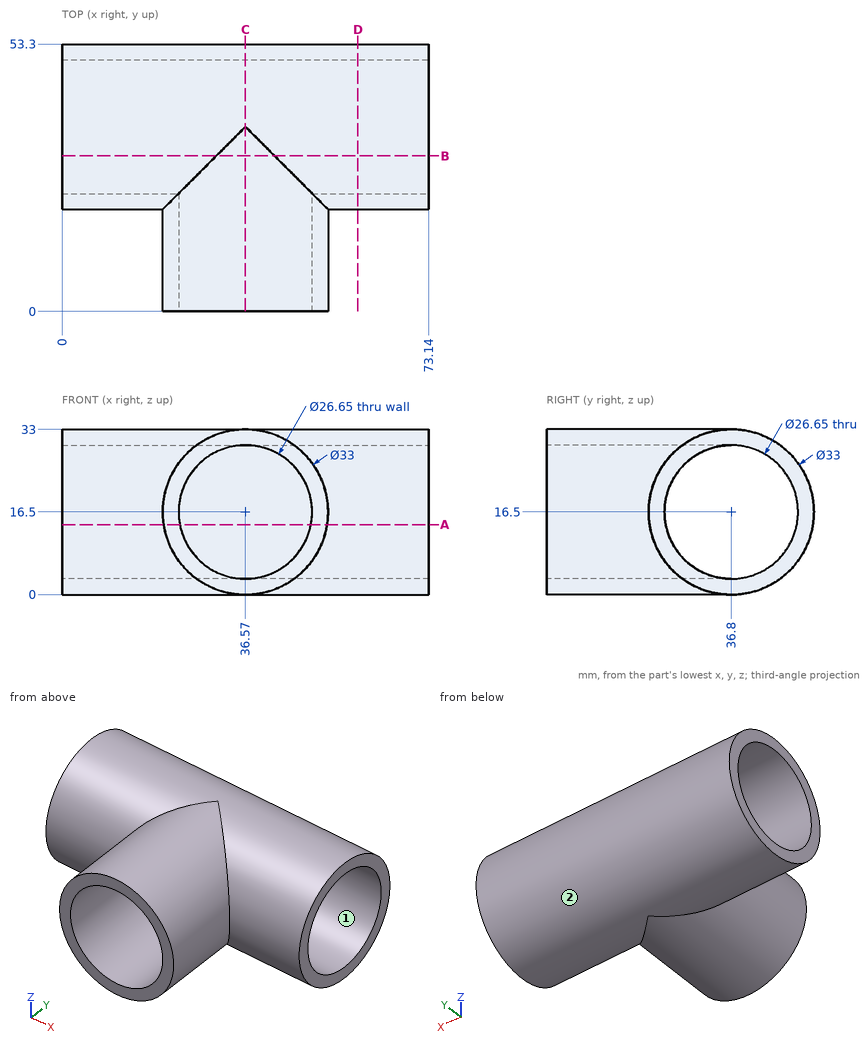
Verification items for this drawing (mm, ordinates from the low corner). Round coordinates to 2 decimals unless told otherwise and drop trailing zeros. Write each loop counter-clockwise with the first axis right and the second up, starting at its lowest first coordinate (ties: lowest second). Pieces come first, ordered by that corner, then holes. Notation, with made-up numbers: (76.25, -17) - (133.25, -17) arc R18 ccw to (133.25, -12) - close; hole circle Ø1 at (24.5, -19). An arc over 180 degrees is marked (long way). Answer as a JSON object with one key per item and string values. Group by question number.
Q1. Thickness scan on line 1 (Z direction, x = 36, y = 23); line 2 (Y direction, x = 7.5, z = 16.5) (3 decimals); line 3 (X direction, y = 10.5, z = 16.5) (3 decimals). Record the ranges inside material, lowest first.
Q2. Mould release check, pull along Z, two halves, no side actions. Record for the marked faces 1 and 2: released by +Z, released by -Z, zero draft, split by the parting line, or undercut.
Q3. Section check C-C, the plane x = 36.57. Enter the section's corners in (y, z) (3 decimals).
Q4. Section check D-D, the plane x = 59. Enter the section's corners in (y, z) (3 decimals).
Q5. Section check A-A, the plane z = 14. Enter the section's corners in (x, y).
Q6. Go/stop test with flat-tipped pins: pin 1 Ø1 at (y, z) = (13, 26) entering from +X; pin 2 Ø1.5 at (x, y) = (55, 24) entering from -Z; pin 3 Ø4 at (x, z) = (59.5, 6.5) entering from +Y. Record where each tip stops, or that it passes through.
Q7. Section check B-B, the plane y = 31. Enter the section's corners in (x, z) (3 decimals).
Found:
{
 "1": {"line 1": "z = 0.01 to 3.19, 29.81 to 32.99", "line 2": "y = 20.3 to 23.475, 50.125 to 53.3", "line 3": "x = 20.07 to 23.245, 49.895 to 53.07"},
 "2": {"face 1": "undercut", "face 2": "split by the parting line"},
 "3": {"outline": "(0, 0) - (36.8, 0) arc R16.5 ccw to (36.8, 33) - (0, 33) - (0, 29.825) - (36.8, 29.825) arc R13.325 cw to (36.8, 3.175) - (0, 3.175) - close"},
 "4": {"outline": "circle Ø33 at (36.8, 16.5); hole circle Ø26.65 at (36.8, 16.5)"},
 "5": {"outline": "(0, 20.49) - (20.26, 20.49) - (20.26, 0) - (23.48, 0) - (23.48, 23.71) - (0, 23.71) - close; (0, 49.89) - (73.14, 49.89) - (73.14, 53.11) - (0, 53.11) - close; (49.66, 0) - (52.88, 0) - (52.88, 20.49) - (73.14, 20.49) - (73.14, 23.71) - (49.66, 23.71) - close"},
 "6": {"pin 1": "stops at x = 50.4", "pin 2": "stops at z = 5.23", "pin 3": "stops at y = 51.23"},
 "7": {"outline": "(0, 1.053) - (30.77, 1.053) arc R16.5 ccw to (42.37, 1.053) - (73.14, 1.053) - (73.14, 4.504) - (42.37, 4.504) arc R13.325 cw to (30.77, 4.504) - (0, 4.504) - close; (0, 28.496) - (30.77, 28.496) arc R13.325 cw to (42.37, 28.496) - (73.14, 28.496) - (73.14, 31.947) - (42.37, 31.947) arc R16.5 ccw to (30.77, 31.947) - (0, 31.947) - close"}
}
